Autodesk Fusion 360 part; units mm, degrees
sketch "Sketch1" plane through (0, 0, 0) normal (0, 0, 1) x (1, 0, 0)
  line L0 (0, 0) -> (126.7, 0)
  line L1 (126.7, 0) -> (126.7, 88.9)
  line L2 (126.7, 88.9) -> (0, 88.9)
  line L3 (0, 88.9) -> (0, 0)
  line L4 (0, 44.45) -> (126.7, 44.45) construction
  line L5 (63.35, 88.9) -> (63.35, 0) construction
  line L6 (4, 84.9) -> (122.7, 84.9)
  line L7 (122.7, 84.9) -> (122.7, 4)
  line L8 (122.7, 4) -> (4, 4)
  line L9 (4, 4) -> (4, 84.9)
  line L10 (4, 84.9) -> (122.7, 4) construction
  line L11 (122.7, 84.9) -> (4, 4) construction
  line L12 (4, 84.9) -> (16, 84.9)
  line L13 (16, 84.9) -> (16, 72.9)
  line L14 (16, 72.9) -> (4, 72.9)
  line L15 (4, 72.9) -> (4, 84.9)
  line L16 (4, 4) -> (16, 4)
  line L17 (16, 4) -> (16, 16)
  line L18 (16, 16) -> (4, 16)
  line L19 (4, 16) -> (4, 4)
  line L20 (122.7, 4) -> (110.7, 4)
  line L21 (110.7, 4) -> (110.7, 16)
  line L22 (110.7, 16) -> (122.7, 16)
  line L23 (122.7, 16) -> (122.7, 4)
  line L24 (122.7, 84.9) -> (110.7, 84.9)
  line L25 (110.7, 84.9) -> (110.7, 72.9)
  line L26 (110.7, 72.9) -> (122.7, 72.9)
  line L27 (122.7, 72.9) -> (122.7, 84.9)
  point P0 (63.35, 44.45)
  dimension "d179" = 126.7
  dimension "d180" = 88.9
  dimension "d181" = 118.7
  dimension "d182" = 80.9
  dimension "d183" = 12
  dimension "d184" = 12
  dimension "d185" = 12
  dimension "d186" = 12
  dimension "d187" = 12
  dimension "d188" = 12
  dimension "d189" = 12
  dimension "d190" = 12
  dimension "d209" = 0
  dimension "d210" = 0
  dimension "d211" = 0
  dimension "d212" = 0
extrude "Extrude1" add sketch "Sketch1" along normal blind 4 contours L6 L7 L8 L9 L13 L14 L17 L18 L21 L22 L25 L26
extrude "Extrude2" add sketch "Sketch1" along normal blind 2 contours L0 L1 L2 L3 | L6 L9 L12 L13 L14 L15 | L6 L7 L24 L25 L26 L27 | L8 L9 L16 L17 L18 L19 | L7 L8 L20 L21 L22 L23
sketch "Sketch2" plane through (0, 0, 0) normal (0, 0, 1) x (1, 0, 0)
  line L0 (126.7, 88.9) -> (0, 88.9)
  line L1 (0, 0) -> (126.7, 0)
  line L2 (117.7, 88.9) -> (117.7, 0) construction
  line L3 (9, 0) -> (9, 88.9) construction
  line L4 (0, 88.9) -> (0, 0)
  line L5 (126.7, 0) -> (126.7, 88.9)
  line L6 (0, 79.9) -> (126.7, 79.9) construction
  line L7 (0, 9) -> (126.7, 9) construction
  line L8 (0, 88.9) -> (0, 0)
  circle A0 centre (9, 9) radius 1.5875
  circle A1 centre (117.7, 9) radius 1.5875
  circle A2 centre (117.7, 79.9) radius 1.5875
  circle A3 centre (9, 79.9) radius 1.5875
  dimension "d195" = 9
  dimension "d196" = 9
  dimension "d197" = 9
  dimension "d198" = 9
  dimension "d199" = 3.175
  dimension "d200" = 3.175
  dimension "d201" = 3.175
  dimension "d202" = 3.175
extrude "Extrude3" cut sketch "Sketch2" along normal blind 10 contours A0 | A1 | A2 | A3
fillet "Fillet1" radius 1 12 edges at (63.35, 84.9, 4) (16, 78.9, 4) (10, 72.9, 4) (4, 44.45, 4) (10, 16, 4) (16, 10, 4) (63.35, 4, 4) (110.7, 10, 4) (116.7, 16, 4) (122.7, 44.45, 4) (116.7, 72.9, 4) (110.7, 78.9, 4)
fillet "Fillet2" radius 1.5 4 edges at (63.35, 88.9, 0) (0, 44.45, 0) (63.35, 0, 0) (126.7, 44.45, 0)
chamfer "Chamfer1" distance 3 angle 30 4 edges at (7.5199, 79.3259, 0) (7.5199, 8.4259, 0) (116.2199, 8.4259, 0) (116.2199, 79.3259, 0) measured on face at (81.0168, 32.9119, 0) measured on face at (81.0168, 32.9119, 0) measured on face at (81.0168, 32.9119, 0) measured on face at (81.0168, 32.9119, 0)
fillet "Fillet3" radius 1 8 edges at (0.4393, 0.4393, 0.4393) (0, 0, 1.75) (0.4393, 88.4607, 0.4393) (0, 88.9, 1.75) (126.2607, 88.4607, 0.4393) (126.7, 88.9, 1.75) (126.2607, 0.4393, 0.4393) (126.7, 0, 1.75)
equation "d181 = 126.7 mm - 8 mm"
equation "d182 = 88.9 mm - 8 mm"
equation "d199 = ( 0.125 * 25.4 ) * 1 mm"
Could you check a few things on this model? Use its own coordinates, in mm. Give positions to 0.01 mm unless a question says otherwise; leave off trailing zeros. Order: outer loops, then holes, each group sorted by start corner. A loop starts at its lowest first (then second) coordinate and runs counter-clockwise, first axis right, second up. Notation, with made-up numbers: (14, 75.25) -> (56, 75.25) arc R9 cw to (56, 81.25) -> close; hole circle Ø4 at (6, 30). An arc over 180 degrees is marked (long way). Return JSON: item names as keys, results as strings.
1. For pin 1 Ø0.8 at (y, z) = (10.5, 2.5) entering from +X; pin 2 Ø2.5 at (x, y) = (9, 9) entering from +Z; pin 3 Ø0.8 at (x, z) = (115, 2.5) entering from -Y; pin 4 Ø1 at (x, z) = (69, 0.5) entering from -Y, each with a flat end and sliding along its axis, tell me the tip position at first contact or that it passes through.
Answer list:
{"pin 1": "stops at x = 110.7", "pin 2": "passes through", "pin 3": "stops at y = 16", "pin 4": "stops at y = 0.09"}
2. Imagine slicing it at A-A on x = 9. List the corners of the cut face in (y, z) for me, then the cut area to 3 significant figures.
Answer list:
{"outline": "(0, 1.5) arc R1.5 ccw to (1.5, 0) -> (4.41, 0) -> (7.41, 1.73) -> (7.41, 2) -> (0, 2) -> close; (10.59, 1.73) -> (13.59, 0) -> (75.31, 0) -> (78.31, 1.73) -> (78.31, 2) -> (72.9, 2) -> (72.9, 3) arc R1 ccw to (71.9, 4) -> (17, 4) arc R1 ccw to (16, 3) -> (16, 2) -> (10.59, 2) -> close; (81.49, 1.73) -> (84.49, 0) -> (87.4, 0) arc R1.5 ccw to (88.9, 1.5) -> (88.9, 2) -> (81.49, 2) -> close", "area": "267 mm2"}
3. I need wall thicknesses on line 1 (X direction, y = 9, z = 1.95); line 2 (Y direction, x = 117.7, z = 1.8); line 3 (X direction, y = 24, z = 3). Which ranges of each line are inside material? Lowest first, please. Write a range as from..to.
Answer list:
{"line 1": "x = 0..7.41, 10.59..116.11, 119.29..126.7", "line 2": "y = 0..7.41, 10.59..78.31, 81.49..88.9", "line 3": "x = 4..122.7"}
4. Imagine slicing it at C-C on x = 22.5. List the corners of the cut face in (y, z) for me, then the cut area to 3 significant figures.
Answer list:
{"outline": "(0, 1.5) arc R1.5 ccw to (1.5, 0) -> (87.4, 0) arc R1.5 ccw to (88.9, 1.5) -> (88.9, 2) -> (84.9, 2) -> (84.9, 3) arc R1 ccw to (83.9, 4) -> (5, 4) arc R1 ccw to (4, 3) -> (4, 2) -> (0, 2) -> close", "area": "338 mm2"}
5. Thinking about a two-plate mould opening in Y: for faces 1 (the flat face through (63, 45, 4)), 2 (the conical face through (7.227, 8.922, 1.624)), which applies, pulls with the +Y half, pulls with the -Y half, needs draft (parallel to the pull), parting line crosses it, or undercut?
Answer list:
{"face 1": "needs draft", "face 2": "undercut"}
6. Imagine slicing it at B-B on y = 79.9. List the corners of the cut face in (x, z) for me.
Answer list:
{"outline": "(0, 1.5) arc R1.5 ccw to (1.5, 0) -> (4.41, 0) -> (7.41, 1.73) -> (7.41, 2) -> (0, 2) -> close; (10.59, 1.73) -> (13.59, 0) -> (113.11, 0) -> (116.11, 1.73) -> (116.11, 2) -> (110.7, 2) -> (110.7, 3) arc R1 ccw to (109.7, 4) -> (17, 4) arc R1 ccw to (16, 3) -> (16, 2) -> (10.59, 2) -> close; (119.29, 1.73) -> (122.29, 0) -> (125.2, 0) arc R1.5 ccw to (126.7, 1.5) -> (126.7, 2) -> (119.29, 2) -> close"}
7. Imagine slicing it at D-D on y = 56. List the corners of the cut face in (x, z) for me, then the cut area to 3 significant figures.
Answer list:
{"outline": "(0, 1.5) arc R1.5 ccw to (1.5, 0) -> (125.2, 0) arc R1.5 ccw to (126.7, 1.5) -> (126.7, 2) -> (122.7, 2) -> (122.7, 3) arc R1 ccw to (121.7, 4) -> (5, 4) arc R1 ccw to (4, 3) -> (4, 2) -> (0, 2) -> close", "area": "489 mm2"}
